from build123d import *

# Parameters (mm, degrees)
SKETCH1_R           = 1.5
SKETCH1_R_2         = 11
SKETCH1_R_3         = 2
BOSS_EXTRUDE1_DEPTH = 5


with BuildPart() as part:
    # Sketch1 → Boss-Extrude1 (new body)
    with BuildSketch(Plane(origin=(0, 0, 0), x_dir=(1, 0, 0), z_dir=(0, 1, 0))):
        with BuildLine():
            ThreePointArc((14.750626914, -58.158567775), (9.981753959, -61.596635254), (8.850376149, -67.3657289))
            ThreePointArc((8.850376149, -67.3657289), (0, -78), (-8.850376149, -67.3657289))
            ThreePointArc((-8.850376149, -67.3657289), (-9.981753959, -61.596635254), (-14.750626914, -58.158567775))
            ThreePointArc((-14.750626914, -58.158567775), (-42.426406871, -42.426406871), (-58.158567775, -14.750626914))
            ThreePointArc((-58.158567775, -14.750626914), (-61.596635254, -9.981753959), (-67.3657289, -8.850376149))
            ThreePointArc((-67.3657289, -8.850376149), (-78, 0), (-67.3657289, 8.850376149))
            ThreePointArc((-67.3657289, 8.850376149), (-61.596635254, 9.981753959), (-58.158567775, 14.750626914))
            ThreePointArc((-58.158567775, 14.750626914), (-42.426406871, 42.426406871), (-14.750626914, 58.158567775))
            ThreePointArc((-14.750626914, 58.158567775), (-9.981753959, 61.596635254), (-8.850376149, 67.3657289))
            ThreePointArc((-8.850376149, 67.3657289), (0, 78), (8.850376149, 67.3657289))
            ThreePointArc((8.850376149, 67.3657289), (9.981753959, 61.596635254), (14.750626914, 58.158567775))
            ThreePointArc((14.750626914, 58.158567775), (42.426406871, 42.426406871), (58.158567775, 14.750626914))
            ThreePointArc((58.158567775, 14.750626914), (61.596635254, 9.981753959), (67.3657289, 8.850376149))
            ThreePointArc((67.3657289, 8.850376149), (78, 0), (67.3657289, -8.850376149))
            ThreePointArc((67.3657289, -8.850376149), (61.596635254, -9.981753959), (58.158567775, -14.750626914))
            ThreePointArc((58.158567775, -14.750626914), (42.426406871, -42.426406871), (14.750626914, -58.158567775))
        make_face()
        with Locations((0, -69)):
            Circle(SKETCH1_R, mode=Mode.SUBTRACT)
        with Locations((-69, 0)):
            Circle(SKETCH1_R, mode=Mode.SUBTRACT)
        with Locations((0, 69)):
            Circle(SKETCH1_R, mode=Mode.SUBTRACT)
        with Locations((69, 0)):
            Circle(SKETCH1_R, mode=Mode.SUBTRACT)
        Circle(SKETCH1_R_2, mode=Mode.SUBTRACT)
        with Locations((9.899494937, 9.899494937)):
            Circle(SKETCH1_R, mode=Mode.SUBTRACT)
        with Locations((9.899494937, -9.899494937)):
            Circle(SKETCH1_R, mode=Mode.SUBTRACT)
        with Locations((-9.899494937, -9.899494937)):
            Circle(SKETCH1_R, mode=Mode.SUBTRACT)
        with Locations((-9.899494937, 9.899494937)):
            Circle(SKETCH1_R, mode=Mode.SUBTRACT)
        with Locations((28.284271247, 28.284271247)):
            Circle(SKETCH1_R_3, mode=Mode.SUBTRACT)
        with Locations((28.284271247, -28.284271247)):
            Circle(SKETCH1_R_3, mode=Mode.SUBTRACT)
        with Locations((-28.284271247, -28.284271247)):
            Circle(SKETCH1_R_3, mode=Mode.SUBTRACT)
        with Locations((-28.284271247, 28.284271247)):
            Circle(SKETCH1_R_3, mode=Mode.SUBTRACT)
    extrude(amount=BOSS_EXTRUDE1_DEPTH)


solid = part.part
The listing builds one solid part. Answer for the finished solid, in the listing's coordinates (mm). Coordinates: 2 decimals unless noted, no trailing zeros. Write each loop counter-clockwise with the first axis right and the second up, starting at its lowest first coordinate (ties: lowest second). Pieces come first, ordered by that corner, then holes. Notation, with made-up numbers: M 57.5,84.5 L 61.5,84.5 A34 ccw 61.5,118.5 Z; hole C -30.75,57.5 d4. An arc over 180 degrees is marked long. Use one line per item in the form item = value.
Item 1: The mould has two halves that part along Z. Classify faces 1 (the face through (18, 5, -1)), 2 (the face through (-61.526, 2.465, 10.028)), 3 (the face through (-9.937, 2.465, 61.668)): released by +Z, released by -Z, zero draft, split by the parting line, or undercut.
Model answer:
face_1 = zero draft
face_2 = released by +Z
face_3 = undercut
Item 2: Given P1, Ø1.8, axis at x = -69, z = 0, coming from the -Y side; P2, Ø3, axis at y = 2, z = 25.5, coming from the +X side, each flat-ended and moving along its own axis, determine where each tip first touches the part or whether it passes through.
Model answer:
P1 = through
P2 = 54.99
Item 3: Find section C-C, the plane z = 22. Give the vertices of the cut face in (x, y).
Model answer:
outline = M -55.82,0 L 55.82,0 L 55.82,5 L -55.82,5 Z
Item 4: Find the intervals of material crossed by probe 1 along Z at (x, y) = (0, 2.8); probe 2 along X at (y, z) = (2.05, 69), in increasing order.
Model answer:
probe_1 = -78 to -70.5, -67.5 to -11, 11 to 67.5, 70.5 to 78
probe_2 = -9 to -1.5, 1.5 to 9
Item 5: Find section B-B, the plane y = 2.5. Give the number of separate pieces and of enclosed holes in the cut face, plus the area to 3 significant figures.
Model answer:
separate_pieces = 1
enclosed_holes = 13
area = 12,000 mm2
Item 6: Find section A-A, the plane z = -4.5. Give the vertices of the cut face in (x, y).
Model answer:
outline = M -76.79,0 L -10.04,0 L -10.04,5 L -76.79,5 Z; M 10.04,0 L 76.79,0 L 76.79,5 L 10.04,5 Z
Item 7: Find section D-D, the plane x = -47. Give the vertices of the cut face in (y, z).
Model answer:
outline = M 0,-37.3 L 5,-37.3 L 5,37.3 L 0,37.3 Z
